Here's how the part is built. I have some questions about the finished solid (model axes, mm). Face numbers are marked on the shaded views. Round coordinates to 2 decimals unless told otherwise and drop trailing zeros. Write each loop counter-clockwise with the first axis right and the second up, starting at its lowest first coordinate (ties: lowest second). Pieces come first, ordered by that corner, then holes. Notation, with made-up numbers: (85, 24) -> (98, 24) arc R18 ccw to (98, 36) -> close; hole circle Ø3 at (75, 59). An arc over 180 degrees is marked (long way). Put each result on its own line as item: value. Start each with the question number.
1) I want a section at C-C, the plane y = -15.25. List the corners of the cut face in (x, z) for me.
2) I want a section at B-B, the plane z = 0. List the corners of the cut face in (x, y) for me.
3) Will these pins go through, and if not, where does the flat tip stop? P1, Ø3, axis at y = -7.5, z = -9, coming from the -X side; P2, Ø3, axis at y = -15, z = 16.5, coming from the -X side; P3, Ø1, axis at y = -8, z = 11, coming from the +X side; P4, Ø6, axis at x = 9, z = -14, coming from the -Y side.
4) If I drill on line 1 along Z through (x, y) = (0, -11.5); line 2 along Y through (x, z) = (9.5, 13); line 3 along Z through (x, y) = (0, -20.65), over which ranges is the centre line in solid material (lowest first)? Write a range as [from, to].
5) I want a section at A-A, the plane x = 0. List the corners of the cut face in (y, z) for me, then the cut area to 3 significant figures.
6) We'd pull the mould along Z, two halves only. Please class the marked faces 1, 2 and 3: released by +Z, released by -Z, zero draft, split by the parting line, or undercut.
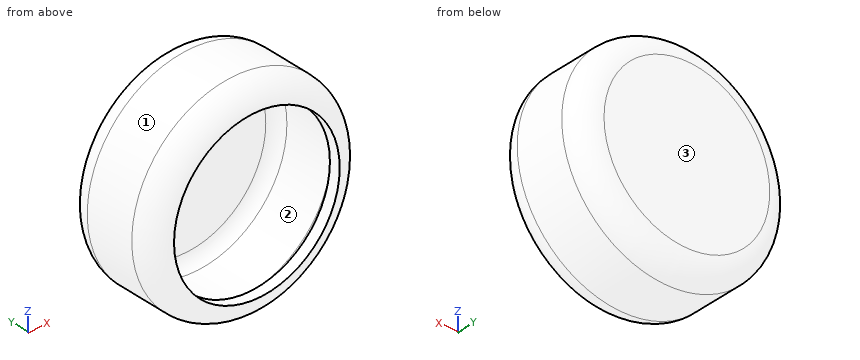
from build123d import *

# Parameters (mm, degrees)
F0_R     = 23.6631657712
F1_DEPTH = 21.69927
F2_R     = 5.08
F3_T     = -2.54


# Not quite as in the source:
# - a shell that OpenCascade refuses in one call is made with other operations: the cavity is built on its own and cut out


with BuildPart() as f1:
    # F0 (on Front) → F1 (new body)
    with BuildSketch(Plane.XZ):
        Circle(F0_R)
    extrude(amount=F1_DEPTH)

    # F2
    f2_edges = [f1.edges().sort_by_distance(p)[0] for p in [
        (-23.663166, -21.69927, 0),
        (-23.663166, 0, 0),
    ]]
    fillet(f2_edges, radius=F2_R)

    # F3: a shell. OpenCascade refuses it in one call, so the cavity is built on its own and cut out:
    # the body offset inwards by the wall thickness, plus a prism from it out through each open face.
    f3_core = offset(f1.part, amount=F3_T, mode=Mode.PRIVATE)
    f3_exits = [f3_core.faces().sort_by_distance(p)[0] for p in [
        (0, -19.15927, 0),
    ]]
    add(f3_core, mode=Mode.SUBTRACT)
    extrude(f3_exits, amount=-F3_T, mode=Mode.SUBTRACT)


solid = f1.part
Findings:
1. outline: circle Ø47.33 at (0, 0); hole circle Ø42.25 at (0, 0)
2. outline: (-23.66, -16.62) arc R5.08 ccw to (-18.58, -21.7) -> (-18.58, -19.16) arc R2.54 cw to (-21.12, -16.62) -> (-21.12, -5.08) arc R2.54 cw to (-18.58, -2.54) -> (18.58, -2.54) arc R2.54 cw to (21.12, -5.08) -> (21.12, -16.62) arc R2.54 cw to (18.58, -19.16) -> (18.58, -21.7) arc R5.08 ccw to (23.66, -16.62) -> (23.66, -5.08) arc R5.08 ccw to (18.58, 0) -> (-18.58, 0) arc R5.08 ccw to (-23.66, -5.08) -> close
3. P1: stops at x = -22.44
3. P2: stops at x = -18.3
3. P3: stops at x = 21.21
3. P4: stops at y = -21.7
4. line 1: z = [-23.66, -21.12], [21.12, 23.66]
4. line 2: y = [-2.54, 0]
4. line 3: z = [-21.68, -18.58], [18.58, 21.68]
5. outline: (-21.7, -18.58) arc R5.08 ccw to (-16.62, -23.66) -> (-5.08, -23.66) arc R5.08 ccw to (0, -18.58) -> (0, 18.58) arc R5.08 ccw to (-5.08, 23.66) -> (-16.62, 23.66) arc R5.08 ccw to (-21.7, 18.58) -> (-19.16, 18.58) arc R2.54 cw to (-16.62, 21.12) -> (-5.08, 21.12) arc R2.54 cw to (-2.54, 18.58) -> (-2.54, -18.58) arc R2.54 cw to (-5.08, -21.12) -> (-16.62, -21.12) arc R2.54 cw to (-19.16, -18.58) -> close
5. area: 214 mm2
6. face 1: split by the parting line
6. face 2: undercut
6. face 3: zero draft
